```python
from build123d import *

# Parameters (mm, degrees)
SALIENTE_EXTRUIR1_DEPTH = 82
CROQUIS3_W              = 10
CROQUIS3_H              = 25
SALIENTE_EXTRUIR2_DEPTH = 1.5
CROQUIS4_W              = 18.5
CROQUIS4_H              = 16
SALIENTE_EXTRUIR3_DEPTH = 2
CROQUIS5_R              = 14.5
CORTAR_EXTRUIR1_DEPTH   = 87.482953955
CROQUIS13_W             = 7.672796091
CROQUIS13_H             = 18.470403829
CROQUIS13_W_2           = 10
CROQUIS13_H_2           = 13
CROQUIS13_W_3           = 18
CORTAR_EXTRUIR9_DEPTH   = 13
CORTAR_EXTRUIR10_DEPTH  = 2
CROQUIS15_W             = 1.990683477
CROQUIS15_H             = 14
CORTAR_EXTRUIR11_DEPTH  = 60
CROQUIS16_W             = 10.5
CROQUIS16_H             = 66
CORTAR_EXTRUIR12_DEPTH  = 10
CROQUIS19_W             = 6
CROQUIS19_H             = 25
SALIENTE_EXTRUIR7_DEPTH = 7
CROQUIS23_R             = 0.5
CORTAR_EXTRUIR13_DEPTH  = 86.732440329


with BuildPart() as part:
    # Croquis2 → Saliente-Extruir1 (new body)
    with BuildSketch(Plane.XY):
        Polygon((-4.596277774, 11.502403514), (-4.596277774, -1.497596486), (9.903722226, -1.497596486), (9.903722226, -4.497596486), (-4.596277774, -4.497596486), (-8.596277774, -4.497596486), (-8.596277774, 11.502403514), align=None)
    extrude(amount=SALIENTE_EXTRUIR1_DEPTH)

    # Croquis3 → Saliente-Extruir2 (add)
    with BuildSketch(Plane(origin=(0, 11.502403514, 0), x_dir=(1, 0, 0), z_dir=(0, 1, 0))):
        with Locations((-9.596277774, -16.5)):
            Rectangle(CROQUIS3_W, CROQUIS3_H)
        with Locations((-9.596277774, -51.5)):
            Rectangle(CROQUIS3_W, CROQUIS3_H)
    extrude(amount=SALIENTE_EXTRUIR2_DEPTH)

    # Croquis4 → Saliente-Extruir3 (add)
    with BuildSketch(Plane.XY.offset(82)):
        with Locations((0.653722226, 3.502403514)):
            Rectangle(CROQUIS4_W, CROQUIS4_H)
    extrude(amount=SALIENTE_EXTRUIR3_DEPTH)

    # Croquis5 → Cortar-Extruir1 (cut, through all)
    with BuildSketch(Plane(origin=(0, -1.497596486, 0), x_dir=(1, 0, 0), z_dir=(0, 1, 0))):
        with Locations((9.903722226, 0)):
            Circle(CROQUIS5_R)
    extrude(amount=-CORTAR_EXTRUIR1_DEPTH, mode=Mode.SUBTRACT)

    # Croquis13 → Cortar-Extruir9 (cut)
    with BuildSketch(Plane.ZY.offset(8.596277774)):
        with Locations((0.163601954, 2.2672016)):
            Rectangle(CROQUIS13_W, CROQUIS13_H)
        with Locations((34, 5.002403514)):
            Rectangle(CROQUIS13_W_2, CROQUIS13_H_2)
        with Locations((73, 5.002403514)):
            Rectangle(CROQUIS13_W_3, CROQUIS13_H_2)
    extrude(amount=-CORTAR_EXTRUIR9_DEPTH, mode=Mode.SUBTRACT)

    # Croquis14 → Cortar-Extruir10 (cut)
    with BuildSketch(Plane.XY.offset(84)):
        with BuildLine():
            Line((-4.096277774, 11.502403514), (9.903722226, 11.502403514))
            Line((9.903722226, 11.502403514), (9.903722226, -2.497596486))
            ThreePointArc((9.903722226, -2.497596486), (0.00422729, 1.602908577), (-4.096277774, 11.502403514))
        make_face()
    extrude(amount=-CORTAR_EXTRUIR10_DEPTH, mode=Mode.SUBTRACT)

    # Croquis15 → Cortar-Extruir11 (cut)
    with BuildSketch(Plane(origin=(0, 0, 4), x_dir=(-1, 0, 0), z_dir=(0, 0, -1))):
        with Locations((6.596277774, 3.502403514)):
            Rectangle(CROQUIS15_W, CROQUIS15_H)
    extrude(amount=-CORTAR_EXTRUIR11_DEPTH, mode=Mode.SUBTRACT)

    # Croquis16 → Cortar-Extruir12 (cut)
    with BuildSketch(Plane.XZ.offset(4.497596486)):
        with Locations((0.653722226, 49)):
            Rectangle(CROQUIS16_W, CROQUIS16_H)
    extrude(amount=-CORTAR_EXTRUIR12_DEPTH, mode=Mode.SUBTRACT)

    # Croquis19 → Saliente-Extruir7 (add)
    with BuildSketch(Plane.XZ.offset(-11.502403514)):
        with Locations((-11.596277774, 16.5)):
            Rectangle(CROQUIS19_W, CROQUIS19_H)
        with Locations((-11.596277774, 51.5)):
            Rectangle(CROQUIS19_W, CROQUIS19_H)
    extrude(amount=SALIENTE_EXTRUIR7_DEPTH)

    # Croquis23 → Cortar-Extruir13 (cut, symmetric)
    with BuildSketch(Plane.XZ.offset(-4.502403514)):
        with Locations(Location((-11.596277774, 45.25, 0), (0, 0, 270))):
            Circle(CROQUIS23_R)
        with Locations(Location((-11.596277774, 57.75, 0), (0, 0, 270))):
            Circle(CROQUIS23_R)
        with Locations(Location((-11.596277774, 51.5, 0), (0, 0, 270))):
            Circle(CROQUIS23_R)
    cortar_extruir13 = extrude(amount=CORTAR_EXTRUIR13_DEPTH, both=True, mode=Mode.SUBTRACT)

    # Simetría1: Cortar-Extruir13 across plane
    add(cortar_extruir13.mirror(Plane(origin=(0, 0, 34), x_dir=(1, 0, 0), z_dir=(0, 0, -1))), mode=Mode.SUBTRACT)


solid = part.part
```
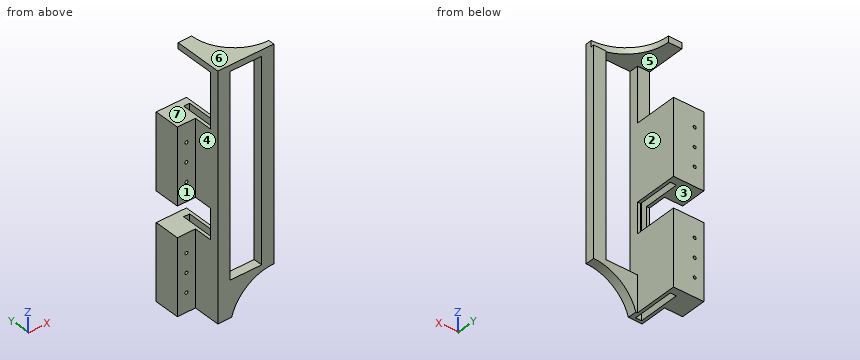
Input: part model. Units: mm. Frame: model coordinates. Face numbers are marked on the shaded views. A direction names the side the tool comes from. Give positions to 0.01 mm unless a question says otherwise; leave off trailing zeros. Order: outer loops, then holes, each group sorted by start corner. A loop starts at its lowest first (then second) coordinate and runs counter-clockwise, first axis right, second up. Notation, with made-up numbers: M 3,-26.5 L 60,-26.5 A21 cw 60,-10.5 Z; hole C 21,33 d2. An arc over 180 degrees is marked long. One line per question, with ' | ' between items. Start each with the question number.
1. Access query for the marked faces 1, 2 and 3. Directions: +Z, -Z, +X, -X, +Y, -Y. A direction counts if a zero-diameter tool reaches every point of the face in a straight line with its end or side. Return the directions, or none.
2. Section query D-D (z = 68). Return the cut outline in (x, y).
3. First-contact query: pin 1 Ø3 at (x, z) = (-6.5, 72.5) entering from +Y; pin 2 Ø3 at (x, z) = (-10.5, 23.5) entering from -Y; pin 3 Ø1.5 at (y, z) = (-3.5, 61) entering from -X; pin 4 Ø7.5 at (x, z) = (-0.5, 52) entering from +Y. Flat tips, straight axial feed; report the tip coordinate or a pass-through.
4. Section query C-C (x = 5). Return the cut outline in (y, z), and give its area (3 significant figures).
5. Pull-direction query (Z, two-part tool) for the marked faces 4, 5, 6 and 7; classes: released by +Z, released by -Z, zero draft, split by the parting line, or undercut.
6. Material intervals for probe 1 along Z at (x, y) = (-8.25, 5.25); probe 2 along X at (y, z) = (8, 10.25); probe 3 along Z at (x, y) = (-9.75, 9.25), sorted ascending. Write a range as [from, to].
7. Section query A-A (z = 59). Return the cut outline in (x, y), and give its area (3 significant figures).
8. Section query B-B (y = 8.5). Count the separate pieces of the cut face and the enclosed holes in it, and give its area (3 significant figures).
Here are the results:
1) face 1: +Z, -Z, -X, -Y | face 2: +Y | face 3: +X, -X, +Y
2) outline: M -8.6,-4.5 L -4.6,-4.5 L -4.6,-1.5 L -8.6,-1.5 Z; M 5.9,-4.5 L 9.9,-4.5 L 9.9,-1.5 L 5.9,-1.5 Z
3) pin 1: y = -1.5 | pin 2: y = 4.5 | pin 3: x = -8.6 | pin 4: through
4) outline: M -4.5,13.65 L -1.5,13.65 L -1.5,16 L -4.5,16 Z; M -4.5,82 L -1.61,82 L -1.61,84 L -4.5,84 Z | area: 12.8 mm²
5) face 4: zero draft | face 5: undercut | face 6: released by +Z | face 7: undercut
6) probe 1: [4, 29], [39, 64], [82, 84] | probe 2: [-14.6, -12.1], [-11.1, -7.59], [-5.6, -4.6] | probe 3: [4, 29], [39, 64]
7) outline: M -14.6,4.5 L -8.6,4.5 L -8.6,-4.5 L -4.6,-4.5 L -4.6,13 L -14.6,13 Z; M 5.9,-4.5 L 9.9,-4.5 L 9.9,-1.5 L 5.9,-1.5 Z; hole M -7.59,-3.5 L -5.6,-3.5 L -5.6,10.5 L -7.59,10.5 Z | area: 105 mm²
8) separate pieces: 5 | enclosed holes: 6 | area: 405 mm²
